Can you work these out from the drawing? Everything is in mm from the part's minimum corner. Round coordinates to 2 decimals unless told otherwise and drop trailing zeros. Loops run counter-clockwise (first coordinate to the right, second up) from the corner with the lowest first, then second, coordinate; pieces in that order, holes last. Notation, with made-up numbers: (71, 63) -> (90, 63) arc R9 ccw to (90, 68) -> close; hole circle Ø1 at (83.5, 32). An arc over 180 degrees is marked (long way). One line per item, written item: value.
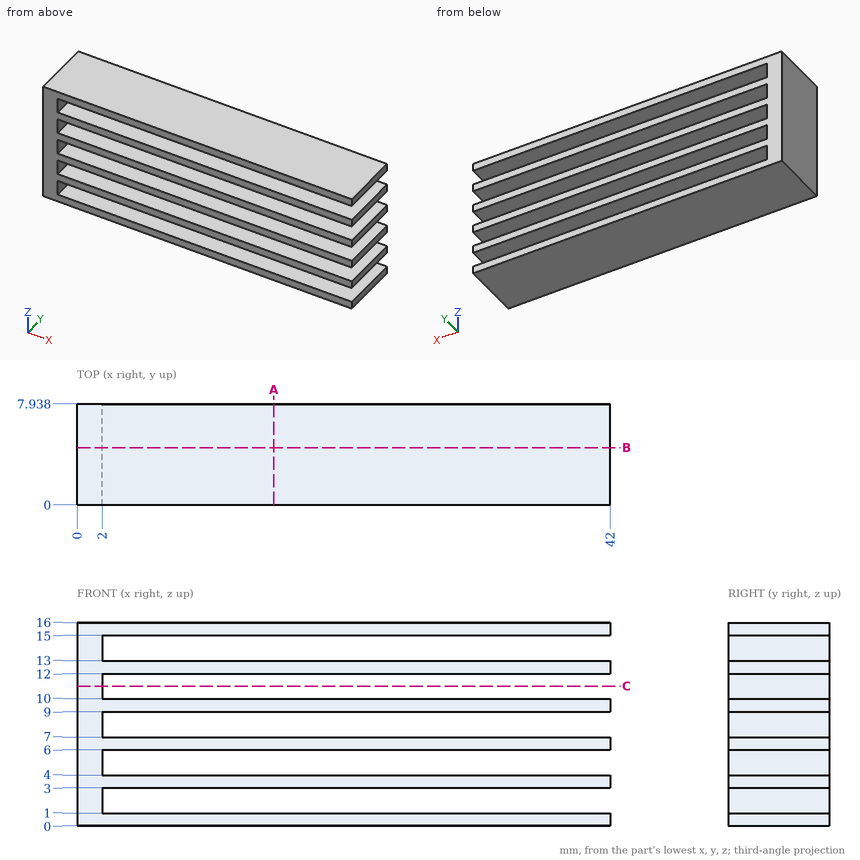
(1) If we section it at B-B, the plane y = 4.5: Please give me the cut outline in (x, z).
Recorded:
outline: (0, 0) -> (42, 0) -> (42, 1) -> (2, 1) -> (2, 3) -> (42, 3) -> (42, 4) -> (2, 4) -> (2, 6) -> (42, 6) -> (42, 7) -> (2, 7) -> (2, 9) -> (42, 9) -> (42, 10) -> (2, 10) -> (2, 12) -> (42, 12) -> (42, 13) -> (2, 13) -> (2, 15) -> (42, 15) -> (42, 16) -> (0, 16) -> close
(2) I'm going to push flat-ended pins straight in: pin 1 Ø4 at (x, y) = (17, 3.5) entering from -Z; pin 2 Ø1.6 at (y, z) = (5, 14) entering from +X. Where does each tip first touch, or does it pass through?
Recorded:
pin 1: z = 0
pin 2: x = 2
(3) If we section it at C-C, the plane z = 11: Please give me the cut outline in (x, y), then the cut area to 3 significant figures.
Recorded:
outline: (0, 0) -> (2, 0) -> (2, 7.94) -> (0, 7.94) -> close
area: 15.9 mm²
(4) If I drill on L1, parallel to Z at x = 11.5, y = 4.5; L2, parallel to X at y = 7.5, z = 1.5, over which ranges is the centre line in solid material (lowest first)?
Recorded:
L1: 0 to 1, 3 to 4, 6 to 7, 9 to 10, 12 to 13, 15 to 16
L2: 0 to 2
(5) If we section it at A-A, the plane x = 15.5: Please give me the cut outline in (y, z).
Recorded:
outline: (0, 0) -> (7.94, 0) -> (7.94, 1) -> (0, 1) -> close; (0, 3) -> (7.94, 3) -> (7.94, 4) -> (0, 4) -> close; (0, 6) -> (7.94, 6) -> (7.94, 7) -> (0, 7) -> close; (0, 9) -> (7.94, 9) -> (7.94, 10) -> (0, 10) -> close; (0, 12) -> (7.94, 12) -> (7.94, 13) -> (0, 13) -> close; (0, 15) -> (7.94, 15) -> (7.94, 16) -> (0, 16) -> close
